Autodesk Inventor part; units mm, degrees
ref_plane "YZ Plane" through (0, 0, 0) normal (1, 0, 0) x (0, 1, 0)
ref_plane "XZ Plane" through (0, 0, 0) normal (0, 1, 0) x (-1, 0, 0)
ref_plane "XY Plane" through (0, 0, 0) normal (0, 0, 1) x (1, 0, 0)
sketch "Sketch1" plane through (0, 0, 0) normal (0, 0, 1) x (1, 0, 0)
  line L0 (0, 0) -> (12.9904, 7.5) construction
  line L1 (0, 0) -> (15, 0) construction
  line L2 (0, 0) -> (-11.3206, 9.8409) construction
  line L3 (0, 0) -> (15, 0) construction
  line L4 (-11.3206, 9.8409) -> (12.9904, 7.5) construction
  line L5 (-11.3206, 9.8409) -> (0, 0)
  line L6 (0, 0) -> (12.9904, 7.5)
  line L7 (12.9904, 7.5) -> (-11.3206, 9.8409)
  line L8 (-11.3206, 9.8409) -> (12.8169, 9.8409) construction
  line L9 (12.8169, 9.8409) -> (12.9904, 7.5) construction
  dimension "d3" = 15
  dimension "d4" = 30
  dimension "d5" = 15
  dimension "d6" = 139
  dimension "d15" = 24.1376
extrude "Extrusion1" add sketch "Sketch1" against normal blind 60
sketch "Sketch4" plane through (0, 0, 0) normal (0, 0, 1) x (1, 0, 0)
  line L0 (-11.3206, 9.8409) -> (12.9904, 7.5)
  line L1 (-11.3206, 9.8409) -> (12.9904, 9.8409)
  line L2 (12.9904, 9.8409) -> (12.9904, 7.5)
  point P0 (0, 0)
extrude "Extrusion4" add sketch "Sketch4" against normal blind 60
sketch "Sketch5" plane through (-11.3206, 9.8409, 0) normal (0, 1, 0) x (1, 0, 0)
  line L0 (24.311, 0) -> (0, 0)
  line L1 (24.311, 0) -> (24.311, 60)
  line L2 (0, 60) -> (24.311, 60)
  line L3 (0, 0) -> (0, 60)
  line L4 (0, 0) -> (0, 60)
  line L5 (0, 30) -> (12.25, 30)
  line L6 (12.25, 30) -> (12.25, 38.89)
  line L7 (11.3206, 0) -> (11.3206, 60)
  line L8 (12.25, 30) -> (21.14, 30) construction
  circle A0 centre (12.25, 38.89) radius 0.95
  line L9 (12.25, 30) -> (12.25, 21.11)
  circle A1 centre (12.25, 21.11) radius 0.95
  dimension "d16" = 12.25
  dimension "d17" = 8.89
  dimension "d18" = 90
  dimension "d19" = 1.9
  dimension "d20" = 8.89
  dimension "d21" = 1.9
extrude "Extrusion5" cut sketch "Sketch5" against normal blind 5 contours A1 L7 | L7 A1 | A0 L7 | L7 A0
sketch "Sketch6" plane through (-11.3206, 9.8409, 0) normal (0, 1, 0) x (1, 0, 0)
  circle A0 centre (12.25, 38.89) radius 0.95
  circle A1 centre (12.25, 21.11) radius 0.95
  line L0 (24.311, 0) -> (0, 0)
  line L1 (24.311, 0) -> (24.311, 60)
  line L2 (0, 60) -> (24.311, 60)
  line L3 (0, 0) -> (0, 60)
  line L4 (11.3206, 0) -> (11.3206, 10)
  line L5 (11.3206, 0) -> (11.3206, 60)
  line L6 (11.3206, 60) -> (11.3206, 50)
  line L7 (0, 0) -> (0, 60)
  line L8 (0, 10) -> (24.311, 10)
  line L9 (0, 50) -> (24.311, 50)
  dimension "d24" = 10
  dimension "d25" = 10
extrude "Extrusion6" cut sketch "Sketch6" against normal blind 20 contours L9 L3 L2 L5 | L5 L2 L1 L9 | L8 L4 L0 L3 | L1 L0 L4 L8
sketch "Sketch7" plane through (-11.3206, 9.8409, -50) normal (0, 1, 0) x (1, 0, 0)
  line L0 (24.311, 0) -> (0, 0)
  line L1 (0, -40) -> (0, 0)
  line L2 (0, -40) -> (24.311, -40)
  line L3 (24.311, -40) -> (24.311, 0)
  circle A0 centre (12.25, -11.11) radius 0.95
  circle A1 centre (12.25, -28.89) radius 0.95
  point P0 (11.3206, -50)
extrude "Extrusion7" add sketch "Sketch7" along normal blind 5.5
properties part number "MirrorMountTest"
The listing builds one solid part. Answer for the finished solid, in the listing's coordinates (mm). A direction names the side the tool comes from. Give positions to 0.01 mm unless a question says otherwise; leave off trailing zeros. Order: outer loops, then holes, each group sorted by start corner. A loop starts at its lowest first (then second) coordinate and runs counter-clockwise, first axis right, second up. Notation, with made-up numbers: (87.25, -13) -> (91.25, -13) arc R5 cw to (91.25, -5) -> close; hole circle Ø8 at (53, 9). An arc over 180 degrees is marked (long way). Write each question's results on one line, items separated by ' | '.
Q1. Which of the six approach directions +Z, -Z, +X, -X, +Y, -Y give full straight-line access (tool end or side, diameter ignored) to faces 5 (the face through (1, 4.841, -21)), 6 (the face through (12.99, 11, -30))?
Checked values:
face 5: +Y | face 6: +Z, -Z, +X, +Y, -Y
Q2. Straight lines are drawn through the part: probe 1 along X at (y, z) = (12, -38.89); probe 2 along X at (y, z) = (8.25, -21); probe 3 along Y at (x, z) = (3.25, -22.5). For each, find the intervals that lie inside material, in ascending order. Write a range as from..to.
Checked values:
probe 1: x = -11.32..-0.02, 1.88..12.99 | probe 2: x = -9.49..-0.01, 1.87..12.99 | probe 3: y = 1.88..15.34
Q3. The part is cut by section D-D, the plane z = -21.11. Give the vertices of the cut face in (x, y), and give its area (3 significant figures).
Checked values:
outline: (-11.32, 9.84) -> (0, 0) -> (12.99, 7.5) -> (12.99, 15.34) -> (1.88, 15.34) -> (1.88, 4.84) -> (-0.02, 4.84) -> (-0.02, 15.34) -> (-11.32, 15.34) -> close | area: 249 mm^2
Q4. The part is cut by section C-C, the plane y = 8.25. Give the vertices of the cut face in (x, z).
Checked values:
outline: (-9.49, -50) -> (12.99, -50) -> (12.99, -10) -> (-9.49, -10) -> close; hole circle Ø1.9 at (0.93, -38.89); hole circle Ø1.9 at (0.93, -21.11)
Q5. Each of these flat-tipped pins is pushed along its axis until it touches: P1, Ø2.5, axis at x = 0.93, z = -21.11, coming from the -Y side; P2, Ø1.5, axis at x = 0.93, z = -38.89, coming from the +Y side; P3, Ø1, axis at x = 2, z = -29.5, coming from the -Y side; P4, Ø5, axis at y = 6.5, z = -41, coming from the -X side. Where does it stop, or does it pass through?
Checked values:
P1: stops at y = 0 | P2: stops at y = 4.84 | P3: stops at y = 0.87 | P4: stops at x = -10.35
Q6. Determine the mould class of faces 1 (the face through (0.806, 10.017, -20.168)), 2 (the face through (-5.74, 4.99, -29.72)), 3 (the face through (1, 15.341, -30)), 4 (the face through (6.404, 3.697, -29.72)) for opening direction X: pulls with the +X half, pulls with the -X half, needs draft (parallel to the pull), parting line crosses it, or undercut.
Checked values:
face 1: undercut | face 2: pulls with the -X half | face 3: needs draft | face 4: pulls with the +X half
Q7. The part is cut by section B-B, the plane x = 1. Give the vertices of the cut face in (y, z), and give its area (3 significant figures).
Checked values:
outline: (0.58, -50) -> (15.34, -50) -> (15.34, -39.84) -> (4.84, -39.84) -> (4.84, -37.94) -> (15.34, -37.94) -> (15.34, -22.06) -> (4.84, -22.06) -> (4.84, -20.16) -> (15.34, -20.16) -> (15.34, -10) -> (0.58, -10) -> close | area: 551 mm^2
Q8. The part is cut by section A-A, the plane z = -31. Give the vertices of the cut face in (x, y), and give its area (3 significant figures).
Checked values:
outline: (-11.32, 9.84) -> (0, 0) -> (12.99, 7.5) -> (12.99, 15.34) -> (-11.32, 15.34) -> close | area: 269 mm^2
